Can you work these out from the drawing? Everything is in mm from the part's minimum corner. Coordinates: 2 decimals unless noted, no trailing zeros. Order: outer loops, then holes, each group sorted by start corner. A loop starts at its lowest first (then second) coordinate and runs counter-clockwise, first axis right, second up. Notation, with made-up numbers: (6, 62) - (40, 62) arc R22 cw to (40, 71) - close; hole circle Ø1 at (-25.75, -22). An arc over 180 degrees is marked (long way). Answer as CSV lines item,"result". Start each with the question number.
Item 1: Imagine slicing it at A-A on z = 2.15. Count the separate pieces of the cut face and the enclosed holes in it, and give its area (3 significant figures).
Item 2: I'm going to push flat-ended pins straight in: pin 1 (2.5 mm diameter, centred on x = 102.5, y = 27.5, fed in from -Z); pin 2 (1 mm diameter, centred on y = 18, z = 3.5, fed in from +X). Where does each tip first touch, or does it pass through?
Item 3: I need wall thicknesses on line 1 (Y direction, x = 80, z = 1.8); line 2 (Y direction, x = 57.5, z = 2.35); line 3 (X direction, y = 4, z = 0.35) (1 decimal). Which ranges of each line are inside material? Lowest first, please.
Item 4: Imagine slicing it at B-B on y = 45. List the corners of the cut face in (x, z) for me.
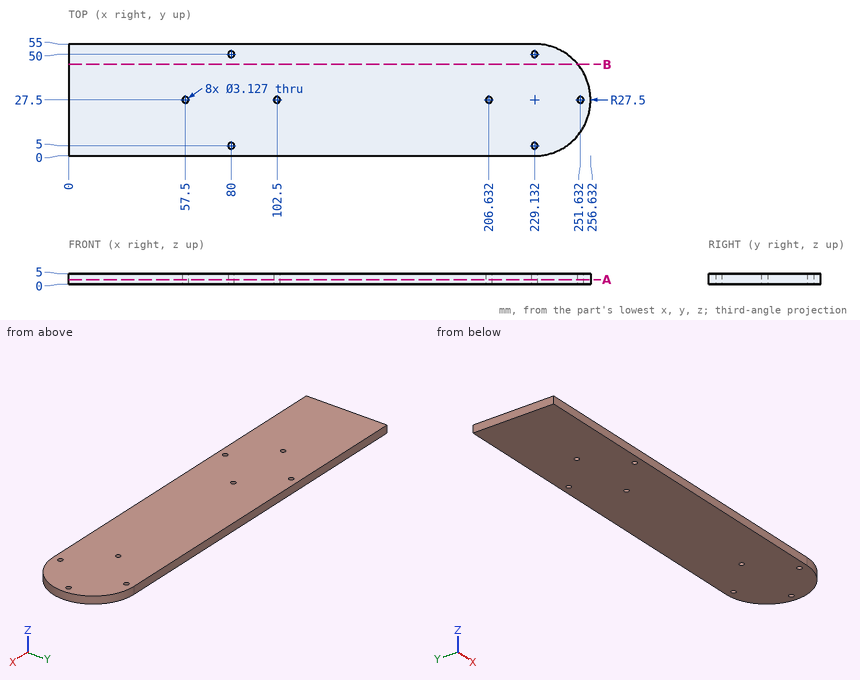
Responses:
1,separate pieces,"1"
1,enclosed holes,"8"
1,area,"13,700 mm^2"
2,pin 1,"passes through"
2,pin 2,"stops at x = 255.12"
3,line 1,"y = 0 to 3.44, 6.56 to 48.44, 51.56 to 55"
3,line 2,"y = 0 to 25.94, 29.06 to 55"
3,line 3,"x = 0 to 78.8, 81.2 to 227.9, 230.3 to 243.4"
4,outline,"(0, 0) - (250.35, 0) - (250.35, 5) - (0, 5) - close"
